from build123d import *

# Parameters (mm, degrees)
SALIENTE_EXTRUIR1_DEPTH = 6


with BuildPart() as part:
    # Croquis1 → Saliente-Extruir1 (new body)
    with BuildSketch(Plane.XY):
        with BuildLine():
            ThreePointArc((7.230331915, -10.196680852), (-10.590936603, -6.639432345), (-6.027091132, 10.950989567))
            Line((-6.027091132, 10.950989567), (16.504287144, 23.351573949))
            ThreePointArc((16.504287144, 23.351573949), (21.353423494, 24.122551849), (25.581793113, 21.626671118))
            Line((25.581793113, 21.626671118), (36.920390006, 7.947353866))
            ThreePointArc((36.920390006, 7.947353866), (40, 6.5), (43.079609994, 7.947353866))
            Line((43.079609994, 7.947353866), (54.418206887, 21.626671118))
            ThreePointArc((54.418206887, 21.626671118), (58.646576506, 24.122551849), (63.495712856, 23.351573949))
            Line((63.495712856, 23.351573949), (86.027091132, 10.950989567))
            ThreePointArc((86.027091132, 10.950989567), (90.590936603, -6.639432345), (72.769668085, -10.196680852))
            Line((72.769668085, -10.196680852), (57.313706213, 0.762937873))
            ThreePointArc((57.313706213, 0.762937873), (54.034506659, 1.381729332), (51.427293643, -0.701175581))
            Line((51.427293643, -0.701175581), (45.180424217, -13.108295407))
            ThreePointArc((45.180424217, -13.108295407), (40, -16.3), (34.819575783, -13.108295407))
            Line((34.819575783, -13.108295407), (28.572706357, -0.701175581))
            ThreePointArc((28.572706357, -0.701175581), (25.965493341, 1.381729332), (22.686293787, 0.762937873))
            Line((22.686293787, 0.762937873), (7.230331915, -10.196680852))
        make_face()
        with BuildLine():
            Line((35.712752372, -12.658589302), (29.465882946, -0.251469477))
            ThreePointArc((29.465882946, -0.251469477), (26.206866677, 2.352161665), (22.107867234, 1.578672341))
            Line((22.107867234, 1.578672341), (6.651905362, -9.380946384))
            ThreePointArc((6.651905362, -9.380946384), (-9.743661675, -6.108277758), (-5.544923841, 10.074910401))
            Line((-5.544923841, 10.074910401), (16.986454434, 22.475494783))
            ThreePointArc((16.986454434, 22.475494783), (21.166744391, 23.140130905), (24.811890615, 20.988509585))
            Line((24.811890615, 20.988509585), (36.150487508, 7.309192332))
            ThreePointArc((36.150487508, 7.309192332), (40, 5.5), (43.849512492, 7.309192332))
            Line((43.849512492, 7.309192332), (55.188109385, 20.988509585))
            ThreePointArc((55.188109385, 20.988509585), (58.833255609, 23.140130905), (63.013545566, 22.475494783))
            Line((63.013545566, 22.475494783), (85.544923841, 10.074910401))
            ThreePointArc((85.544923841, 10.074910401), (89.743661675, -6.108277758), (73.348094638, -9.380946384))
            Line((73.348094638, -9.380946384), (57.892132766, 1.578672341))
            ThreePointArc((57.892132766, 1.578672341), (53.793133323, 2.352161665), (50.534117054, -0.251469477))
            Line((50.534117054, -0.251469477), (44.287247628, -12.658589302))
            ThreePointArc((44.287247628, -12.658589302), (40, -15.3), (35.712752372, -12.658589302))
        make_face(mode=Mode.SUBTRACT)
    extrude(amount=SALIENTE_EXTRUIR1_DEPTH)


solid = part.part
Geometry: final body of the model. Coordinates: model frame, mm. A direction names the side the tool comes from. Coordinates: 2 decimals unless noted, no trailing zeros. Write each loop counter-clockwise with the first axis right and the second up, starting at its lowest first coordinate (ties: lowest second). Pieces come first, ordered by that corner, then holes. Notation, with made-up numbers: (19, -13) - (24, -13) arc R12 cw to (24, -4) - close; hole circle Ø1 at (33.5, -12). An arc over 180 degrees is marked (long way). Return JSON: item names as keys, results as strings.
Item 1: Pin query (flat end, axial travel): pin 1 Ø3 at (x, z) = (24, 1.5) entering from -Y; pin 2 Ø3 at (y, z) = (-2, 5) entering from -X. Return the tip coordinate at first contact, or that it passes through.
Completed:
{"pin 1": "stops at y = 0.63", "pin 2": "stops at x = -12.49"}
Item 2: Reachability of faces 1 (the face through (48.348, -6.818, 2.958)), 2 (the face through (31.172, 14.883, 2.958)), 3 (the face through (26.265, 2.337, 2.958)) from +Z, -Z, +X, -X, +Y, -Y: full face, straight path, thin tool, end or side. Return the list, or none.
Completed:
{"face 1": "+Z, -Z, -Y", "face 2": "+Z, -Z, +Y", "face 3": "+Z, -Z"}
Item 3: Pull-direction query (Y, two-part tool) for faces 4 (the face through (89.88, -5.885, 2.958)), 5 (the face through (65.15, -4.794, 2.958)), 6 (the face through (90.739, -6.396, 2.958)), 7 (the face through (14.488, -3.824, 2.958)); classes: +Y half, -Y half, draft (parallel to the pull), parting line (faces both ways), or undercut.
Completed:
{"face 4": "undercut", "face 5": "-Y half", "face 6": "parting line", "face 7": "undercut"}
Item 4: Line query: L1, parallel to X at y = -9, z = 4.8; L2, parallel to X at y = -7.5, z = 2.05; L3, parallel to X at y = 19.5, z = 2.9. Output: solid intervals per line, ascending.
Completed:
{"L1": "x = -8.67 to -7.16, 7.19 to 8.92, 32.75 to 33.87, 46.13 to 47.25, 71.08 to 72.81, 87.16 to 88.67", "L2": "x = -10 to -8.72, 9.3 to 11.03, 32 to 33.12, 46.88 to 48, 68.97 to 70.7, 88.72 to 90", "L3": "x = 9.51 to 11.58, 26.05 to 27.34, 52.66 to 53.95, 68.42 to 70.49"}
Item 5: Section query A-A (x = 20). Output: boundary loops of the cut face in (y, z), and give its area (3 significant figures).
Completed:
{"outline": "(-1.14, 0) - (0.08, 0) - (0.08, 6) - (-1.14, 6) - close; (23.25, 0) - (24.25, 0) - (24.25, 6) - (23.25, 6) - close", "area": "13.4 mm2"}
Item 6: Section query C-C (y = 19.5). Output: boundary loops of the cut face in (x, z), and give its area (3 significant figures).
Completed:
{"outline": "(9.51, 0) - (11.58, 0) - (11.58, 6) - (9.51, 6) - close; (26.05, 0) - (27.34, 0) - (27.34, 6) - (26.05, 6) - close; (52.66, 0) - (53.95, 0) - (53.95, 6) - (52.66, 6) - close; (68.42, 0) - (70.49, 0) - (70.49, 6) - (68.42, 6) - close", "area": "40.5 mm2"}
Item 7: Section query D-D (y = 4). Output: boundary loops of the cut face in (x, z).
Completed:
{"outline": "(-11.84, 0) - (-10.78, 0) - (-10.78, 6) - (-11.84, 6) - close; (90.78, 0) - (91.84, 0) - (91.84, 6) - (90.78, 6) - close"}
